from build123d import *

# Parameters (mm, degrees)
F0_R     = 2.5
F1_DEPTH = 500


with BuildPart() as f1:
    # F0 (on Right) → F1 (new body)
    with BuildSketch(Plane.YZ):
        with BuildLine():
            Line((-3.1, 15), (-12, 15))
            ThreePointArc((-12, 15), (-14.12132, 14.12132), (-15, 12))
            Line((-15, 12), (-15, 3.1))
            Line((-15, 3.1), (-12.8, 3.1))
            ThreePointArc((-12.8, 3.1), (-12.234315, 3.334315), (-12, 3.9))
            Line((-12, 3.9), (-12, 5.6))
            Line((-12, 5.6), (-13.5, 5.6))
            Line((-13.5, 5.6), (-13.5, 8.15))
            Line((-13.5, 8.15), (-10.805, 8.15))
            ThreePointArc((-10.805, 8.15), (-9.65695, 7.921639), (-8.68368, 7.27132))
            Line((-8.68368, 7.27132), (-6.12868, 4.71632))
            ThreePointArc((-6.12868, 4.71632), (-5.478361, 3.74305), (-5.25, 2.595))
            Line((-5.25, 2.595), (-5.25, -2.595))
            ThreePointArc((-5.25, -2.595), (-5.478361, -3.74305), (-6.12868, -4.71632))
            Line((-6.12868, -4.71632), (-8.68368, -7.27132))
            ThreePointArc((-8.68368, -7.27132), (-9.65695, -7.921639), (-10.805, -8.15))
            Line((-10.805, -8.15), (-13.5, -8.15))
            Line((-13.5, -8.15), (-13.5, -5.6))
            Line((-13.5, -5.6), (-12, -5.6))
            Line((-12, -5.6), (-12, -3.9))
            ThreePointArc((-12, -3.9), (-12.234315, -3.334315), (-12.8, -3.1))
            Line((-12.8, -3.1), (-15, -3.1))
            Line((-15, -3.1), (-15, -12))
            ThreePointArc((-15, -12), (-14.12132, -14.12132), (-12, -15))
            Line((-12, -15), (-3.1, -15))
            Line((-3.1, -15), (-3.1, -12.8))
            ThreePointArc((-3.1, -12.8), (-3.334315, -12.234315), (-3.9, -12))
            Line((-3.9, -12), (-5.6, -12))
            Line((-5.6, -12), (-5.6, -13.5))
            Line((-5.6, -13.5), (-8.15, -13.5))
            Line((-8.15, -13.5), (-8.15, -10.805))
            ThreePointArc((-8.15, -10.805), (-7.921639, -9.65695), (-7.27132, -8.68368))
            Line((-7.27132, -8.68368), (-4.71632, -6.12868))
            ThreePointArc((-4.71632, -6.12868), (-3.74305, -5.478361), (-2.595, -5.25))
            Line((-2.595, -5.25), (2.595, -5.25))
            ThreePointArc((2.595, -5.25), (3.74305, -5.478361), (4.71632, -6.12868))
            Line((4.71632, -6.12868), (7.27132, -8.68368))
            ThreePointArc((7.27132, -8.68368), (7.921639, -9.65695), (8.15, -10.805))
            Line((8.15, -10.805), (8.15, -13.5))
            Line((8.15, -13.5), (5.6, -13.5))
            Line((5.6, -13.5), (5.6, -12))
            Line((5.6, -12), (3.9, -12))
            ThreePointArc((3.9, -12), (3.334315, -12.234315), (3.1, -12.8))
            Line((3.1, -12.8), (3.1, -15))
            Line((3.1, -15), (12, -15))
            ThreePointArc((12, -15), (14.12132, -14.12132), (15, -12))
            Line((15, -12), (15, -3.1))
            Line((15, -3.1), (12.8, -3.1))
            ThreePointArc((12.8, -3.1), (12.234315, -3.334315), (12, -3.9))
            Line((12, -3.9), (12, -5.6))
            Line((12, -5.6), (13.5, -5.6))
            Line((13.5, -5.6), (13.5, -8.15))
            Line((13.5, -8.15), (10.805, -8.15))
            ThreePointArc((10.805, -8.15), (9.65695, -7.921639), (8.68368, -7.27132))
            Line((8.68368, -7.27132), (6.12868, -4.71632))
            ThreePointArc((6.12868, -4.71632), (5.478361, -3.74305), (5.25, -2.595))
            Line((5.25, -2.595), (5.25, 2.595))
            ThreePointArc((5.25, 2.595), (5.478361, 3.74305), (6.12868, 4.71632))
            Line((6.12868, 4.71632), (8.68368, 7.27132))
            ThreePointArc((8.68368, 7.27132), (9.65695, 7.921639), (10.805, 8.15))
            Line((10.805, 8.15), (13.5, 8.15))
            Line((13.5, 8.15), (13.5, 5.6))
            Line((13.5, 5.6), (12, 5.6))
            Line((12, 5.6), (12, 3.9))
            ThreePointArc((12, 3.9), (12.234315, 3.334315), (12.8, 3.1))
            Line((12.8, 3.1), (15, 3.1))
            Line((15, 3.1), (15, 12))
            ThreePointArc((15, 12), (14.12132, 14.12132), (12, 15))
            Line((12, 15), (3.1, 15))
            Line((3.1, 15), (3.1, 12.8))
            ThreePointArc((3.1, 12.8), (3.334315, 12.234315), (3.9, 12))
            Line((3.9, 12), (5.6, 12))
            Line((5.6, 12), (5.6, 13.5))
            Line((5.6, 13.5), (8.15, 13.5))
            Line((8.15, 13.5), (8.15, 10.805))
            ThreePointArc((8.15, 10.805), (7.921639, 9.65695), (7.27132, 8.68368))
            Line((7.27132, 8.68368), (4.71632, 6.12868))
            ThreePointArc((4.71632, 6.12868), (3.74305, 5.478361), (2.595, 5.25))
            Line((2.595, 5.25), (-2.595, 5.25))
            ThreePointArc((-2.595, 5.25), (-3.74305, 5.478361), (-4.71632, 6.12868))
            Line((-4.71632, 6.12868), (-7.27132, 8.68368))
            ThreePointArc((-7.27132, 8.68368), (-7.921639, 9.65695), (-8.15, 10.805))
            Line((-8.15, 10.805), (-8.15, 13.5))
            Line((-8.15, 13.5), (-5.6, 13.5))
            Line((-5.6, 13.5), (-5.6, 12))
            Line((-5.6, 12), (-3.9, 12))
            ThreePointArc((-3.9, 12), (-3.334315, 12.234315), (-3.1, 12.8))
            Line((-3.1, 12.8), (-3.1, 15))
        make_face()
        with BuildLine():
            ThreePointArc((-12, -13.5), (-13.06066, -13.06066), (-13.5, -12))
            Line((-13.5, -12), (-13.5, -9.65))
            Line((-13.5, -9.65), (-9.65, -9.65))
            Line((-9.65, -9.65), (-9.65, -13.5))
            Line((-9.65, -13.5), (-12, -13.5))
        make_face(mode=Mode.SUBTRACT)
        with BuildLine():
            ThreePointArc((13.5, -12), (13.06066, -13.06066), (12, -13.5))
            Line((12, -13.5), (9.65, -13.5))
            Line((9.65, -13.5), (9.65, -9.65))
            Line((9.65, -9.65), (13.5, -9.65))
            Line((13.5, -9.65), (13.5, -12))
        make_face(mode=Mode.SUBTRACT)
        Circle(F0_R, mode=Mode.SUBTRACT)
        with BuildLine():
            ThreePointArc((-13.5, 12), (-13.06066, 13.06066), (-12, 13.5))
            Line((-12, 13.5), (-9.65, 13.5))
            Line((-9.65, 13.5), (-9.65, 9.65))
            Line((-9.65, 9.65), (-13.5, 9.65))
            Line((-13.5, 9.65), (-13.5, 12))
        make_face(mode=Mode.SUBTRACT)
        with BuildLine():
            ThreePointArc((12, 13.5), (13.06066, 13.06066), (13.5, 12))
            Line((13.5, 12), (13.5, 9.65))
            Line((13.5, 9.65), (9.65, 9.65))
            Line((9.65, 9.65), (9.65, 13.5))
            Line((9.65, 13.5), (12, 13.5))
        make_face(mode=Mode.SUBTRACT)
    extrude(amount=F1_DEPTH)


solid = f1.part
Check sheet for the modelled part. Datum: model origin and axes. Units: mm. Round coordinates to 2 decimals unless told otherwise and drop trailing zeros. Answer as CSV lines item,"result". Start each with the question number.
1) Section check A-A on x = 278.5. State how many separate pieces and enclosed holes the cut face has, and give its area (3 significant figures).
2) Material ranges on line 1 (Z direction, x = 398, y = -13.25); line 2 (Z direction, x = 377, y = 7.25); line 3 (Z direction, x = 134, y = 0), recorded low to high. Write a range as from..to.
3) Go/stop test with flat-tipped pins: P1, Ø2.5, axis at x = 216.5, y = -14, coming from the -Z side; P2, Ø1.8, axis at x = 332, y = 14, coming from the -Z side; P3, Ø1.2, axis at x = 262.5, z = 13, coming from the -Y side. Record where each tip stops, or that it passes through.
Found:
1,separate pieces,"1"
1,enclosed holes,"5"
1,area,"347 mm^2"
2,line 1,"z = -14.73..-12.83, -9.65..-8.15, -5.6..-3.1, 3.1..5.6, 8.15..9.65, 12.83..14.73"
2,line 2,"z = -15..-13.5, -8.66..-5.84, 5.84..8.66, 13.5..15"
2,line 3,"z = -5.25..-2.5, 2.5..5.25"
3,P1,"stops at z = -14.9"
3,P2,"stops at z = -14.79"
3,P3,"stops at y = -14.97"
